Source: CAD feature listing. Evaluate the final solid. Frame: model axes, mm. A direction names the side the tool comes from. Round coordinates to 2 decimals unless told otherwise and drop trailing zeros. Write each loop counter-clockwise with the first axis right and the second up, starting at its lowest first coordinate (ties: lowest second). Pieces come first, ordered by that corner, then holes. Notation, with made-up numbers: M 62,84.25 L 121,84.25 A14 cw 121,108.25 Z; hole C 34,15 d1. An arc over 180 degrees is marked long. Use a Markdown table: item, result.
```python
from build123d import *

# Parameters (mm, degrees)
SKIZZE1_W                       = 5
SKIZZE1_H                       = 80
M4_GEWINDEBOHRUNG1_D            = 3.3
M4_GEWINDEBOHRUNG1_DEPTH        = 40
M4_GEWINDEBOHRUNG1_TIP          = 0.991420021
SKIZZE5_W                       = 4.2
SKIZZE5_H                       = 4.2
SCHNITT_LINEAR_AUSTRAGEN1_DEPTH = 10
FASE1_SIZE                      = 1


with BuildPart() as part:
    # Skizze1 → Rotation1 (revolve)
    with BuildSketch(Plane(origin=(0, 0, 0), x_dir=(0, 0, -1), z_dir=(1, 0, 0))):
        with Locations((-2.5, 40)):
            Rectangle(SKIZZE1_W, SKIZZE1_H)
    revolve(axis=Axis((0, 0, 0), (0, -1, 0)))

    # M4 Gewindebohrung1
    with Locations(Plane(origin=(0, 0, 0), x_dir=(-1, 0, 0), z_dir=(0, -1, 0))):
        with Locations((0, 0)):
            Hole(M4_GEWINDEBOHRUNG1_D / 2, depth=M4_GEWINDEBOHRUNG1_DEPTH)
            with Locations((0, 0, -(M4_GEWINDEBOHRUNG1_DEPTH + M4_GEWINDEBOHRUNG1_TIP / 2))):  # 118° drill point
                Cone(0, M4_GEWINDEBOHRUNG1_D / 2, M4_GEWINDEBOHRUNG1_TIP, mode=Mode.SUBTRACT)

    # Skizze5 → Schnitt-Linear austragen1 (cut, symmetric)
    with BuildSketch(Plane.XY):
        with Locations((-5, 17.1)):
            Rectangle(SKIZZE5_W, SKIZZE5_H)
    schnitt_linear_austragen1 = extrude(amount=SCHNITT_LINEAR_AUSTRAGEN1_DEPTH, both=True, mode=Mode.SUBTRACT)

    # Spiegeln1: Schnitt-Linear austragen1 across plane
    add(schnitt_linear_austragen1.mirror(Plane(origin=(0, 0, 0), x_dir=(0, 0, 1), z_dir=(1, 0, 0))), mode=Mode.SUBTRACT)

    # Fase1
    fase1_edges = [part.edges().sort_by_distance(p)[0] for p in [
        (0, 80, -5),
    ]]
    chamfer(fase1_edges, length=FASE1_SIZE)


solid = part.part
```
Q1. Section A-A on y = 38. Return loops of the section in (x, z).
Results are:
| item | result |
|---|---|
| outline | C 0,0 d10; hole C 0,0 d3.3 |
Q2. Section B-B on y = 66. Return loops of the section in (x, z).
Results are:
| item | result |
|---|---|
| outline | C 0,0 d10 |
Q3. Reachability of faces 5 (the flat face through (4, 19.2, 0)), 6 (the flat face through (-4, 15, 0)), 7 (the cylindrical face through (-1.216, 20.28, -1.115)) from +Z, -Z, +X, -X, +Y, -Y: full face, straight path, thin tool, end or side. Return the list, or none.
Results are:
| item | result |
|---|---|
| face 5 | +Z, -Z, +X |
| face 6 | +Z, -Z, -X |
| face 7 | -Y |
Q4. Mould query, pull axis Y, two halves, no side actions, for faces 1 (the flat face through (-4, 19.2, 0)), 2 (the cylindrical face through (4.88, 40.05, -1.08)), 3 (the flat face through (2.9, 17, 0)), 4 (the flat face through (0, 80, 0)). Classes: +Y half, -Y half, draft (parallel to the pull), parting line (faces both ways), or undercut.
Results are:
| item | result |
|---|---|
| face 1 | undercut |
| face 2 | draft |
| face 3 | undercut |
| face 4 | +Y half |
Q5. First-contact query: pin 1 Ø5 at (x, y) = (-4, 28.5) entering from -Z; pin 2 Ø2 at (y, z) = (17.5, -0.5) entering from +X; pin 3 Ø3 at (x, y) = (-2.5, 54) entering from -Z. Flat tips, straight axial feed; report the tip coordinate or a pass-through.
Results are:
| item | result |
|---|---|
| pin 1 | z = -4.77 |
| pin 2 | x = 2.9 |
| pin 3 | z = -4.9 |
Q6. Line query: L1, parallel to Y at x = -3, z = 1.25; L2, parallel to Z at x = 0, y = 28; L3, parallel to X at y = 11, z = -3. Output: solid intervals per line, ascending.
Results are:
| item | result |
|---|---|
| L1 | 0 to 15, 19.2 to 80 |
| L2 | -5 to -1.65, 1.65 to 5 |
| L3 | -4 to 4 |
